Input: dimensioned drawing with shaded views. Units: mm. Origin: part minimum x, y, z. Give positions to 0.01 mm unless a question says otherwise; leave off trailing zeros. Order: outer loops, then holes, each group sorted by start corner. A loop starts at its lowest first (then second) coordinate and runs counter-clockwise, first axis right, second up.
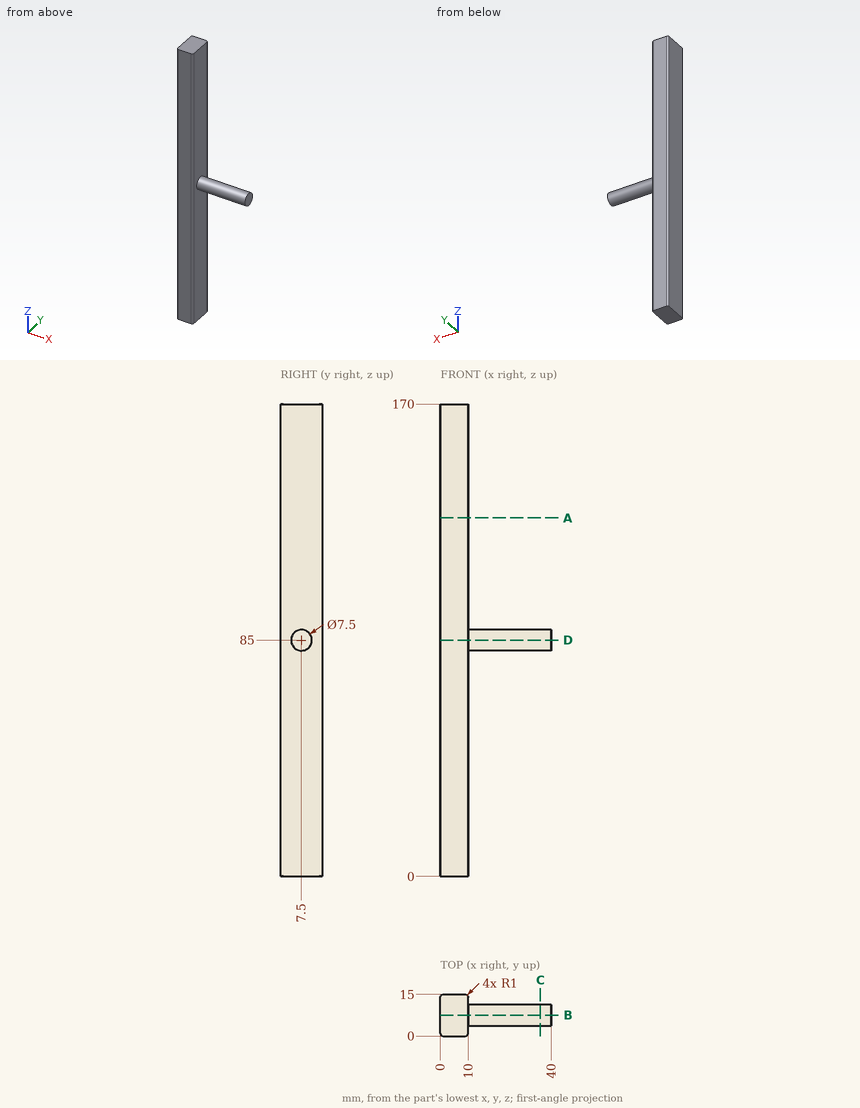
1) Section query C-C, the plane x = 36. Return the cut outline in (y, z).
Report:
outline: circle Ø7.5 at (7.5, 85)
2) Material intervals for L1, parallel to Z at x = 33, y = 7.25; L2, parallel to X at y = 2.5, z = 162; L3, parallel to Z at x = 22, y = 10, sorted ascending.
Report:
L1: z = 81.26 to 88.74
L2: x = 0 to 10
L3: z = 82.2 to 87.8
3) Section query A-A, the plane z = 129. Return the cut outline in (x, y).
Report:
outline: (0, 1) arc R1 ccw to (1, 0) - (9, 0) arc R1 ccw to (10, 1) - (10, 14) arc R1 ccw to (9, 15) - (1, 15) arc R1 ccw to (0, 14) - close
4) Pin query (flat end, axial travel): pin 1 (4 mm diameter, centred on y = 10.5, z = 57.5, fed in from +X); pin 2 (4 mm diameter, centred on x = 17.5, z = 89.5, fed in from +Y); pin 3 (4 mm diameter, centred on x = 29.5, y = 5, fed in from -Z). Return the tip coordinate at first contact, or that it passes through.
Report:
pin 1: stops at x = 10
pin 2: stops at y = 10.3
pin 3: stops at z = 81.28
5) Section query D-D, the plane z = 85. Return the cut outline in (x, y), and give its area (3 significant figures).
Report:
outline: (0, 1) arc R1 ccw to (1, 0) - (9, 0) arc R1 ccw to (10, 1) - (10, 3.75) - (40, 3.75) - (40, 11.25) - (10, 11.25) - (10, 14) arc R1 ccw to (9, 15) - (1, 15) arc R1 ccw to (0, 14) - close
area: 374 mm2
6) Section query B-B, the plane y = 7.5. Return the cut outline in (x, z), and give its area (4 significant figures).
Report:
outline: (0, 0) - (10, 0) - (10, 81.25) - (40, 81.25) - (40, 88.75) - (10, 88.75) - (10, 170) - (0, 170) - close
area: 1,925 mm2
